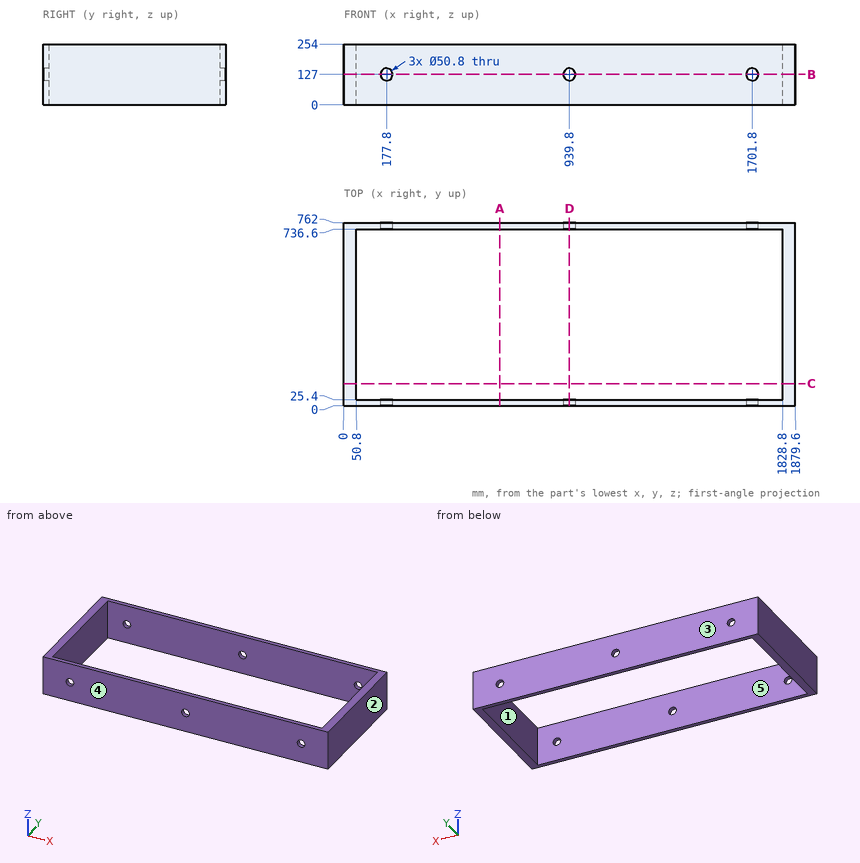
For this review, use the dimensioned drawing (mm, ordinates from the lowest corner) and the shaded views. A direction names the side the tool comes from. Round coordinates to 2 decimals unless told otherwise and drop trailing zeros. Write each loop counter-clockwise with the first axis right and the second up, starting at its lowest first coordinate (ties: lowest second). Pieces come first, ordered by that corner, then holes. Notation, with made-up numbers: (78, 68) - (104, 68) arc R9 ccw to (104, 85) - close; hole circle Ø2 at (70.5, -12). An arc over 180 degrees is marked (long way). Use CSV: the item, a comma, the result in double quotes.
1) The part is to be moulded in two halves that separate along X. For the marked faces 1, 2 and 3, say which applies: pulls with the +X half, pulls with the -X half, needs draft (parallel to the pull), parting line crosses it, or undercut.
Conclusion:
face 1,"undercut"
face 2,"pulls with the +X half"
face 3,"needs draft"
2) Add section C-C on y = 92.5. Write out the cut boundary in (x, z), and give its area (3 significant figures).
Conclusion:
outline,"(0, 0) - (50.8, 0) - (50.8, 254) - (0, 254) - close; (1828.8, 0) - (1879.6, 0) - (1879.6, 254) - (1828.8, 254) - close"
area,"25,800 mm^2"
3) Add section D-D on x = 939.8. Write out the cut boundary in (y, z).
Conclusion:
outline,"(0, 0) - (25.4, 0) - (25.4, 101.6) - (0, 101.6) - close; (0, 152.4) - (25.4, 152.4) - (25.4, 254) - (0, 254) - close; (736.6, 0) - (762, 0) - (762, 101.6) - (736.6, 101.6) - close; (736.6, 152.4) - (762, 152.4) - (762, 254) - (736.6, 254) - close"
4) Add section B-B on z = 127. Count the separate pieces of the cut face and the enclosed holes in it, and give its area (3 significant figures).
Conclusion:
separate pieces,"6"
enclosed holes,"0"
area,"160,000 mm^2"
5) For the marked faces 4 and 5, list the 3-axis set-ups (+Z, -Z, +X, -X, +Y, -Y) from which the entire face can be reached by the end or side of a thin tool; tool diameter is ignored.
Conclusion:
face 4,"+Z, -Z, +X, -X, -Y"
face 5,"+Z, -Z"
6) Wall thickness on line 1 along X through (y, z) = (110, 145.5); line 2 along Y through (x, z) = (952, 13); line 3 along Z through (x, y) = (1701.8, 6.5): over which ranges is each line inside the solid? List them lowest first. Write a range as from..to.
Conclusion:
line 1,"x = 0..50.8, 1828.8..1879.6"
line 2,"y = 0..25.4, 736.6..762"
line 3,"z = 0..101.6, 152.4..254"
7) Add section A-A on x = 650. Write out the cut boundary in (y, z), and give its area (3 significant figures).
Conclusion:
outline,"(0, 0) - (25.4, 0) - (25.4, 254) - (0, 254) - close; (736.6, 0) - (762, 0) - (762, 254) - (736.6, 254) - close"
area,"12,900 mm^2"
